Print and shaded views of the part. All mm, measured from the part's lowest x, y and z. Coordinates: 2 decimals unless noted, no trailing zeros. Loops run counter-clockwise (first coordinate to the right, second up) from the corner with the lowest first, then second, coordinate; pieces in that order, holes last. Notation, with made-up numbers: (8.25, 55) -> (18.25, 55) arc R29 ccw to (18.25, 77) -> close; hole circle Ø2 at (64.25, 44). An arc over 180 degrees is marked (long way). One line per item, written item: value. Start each with the question number.
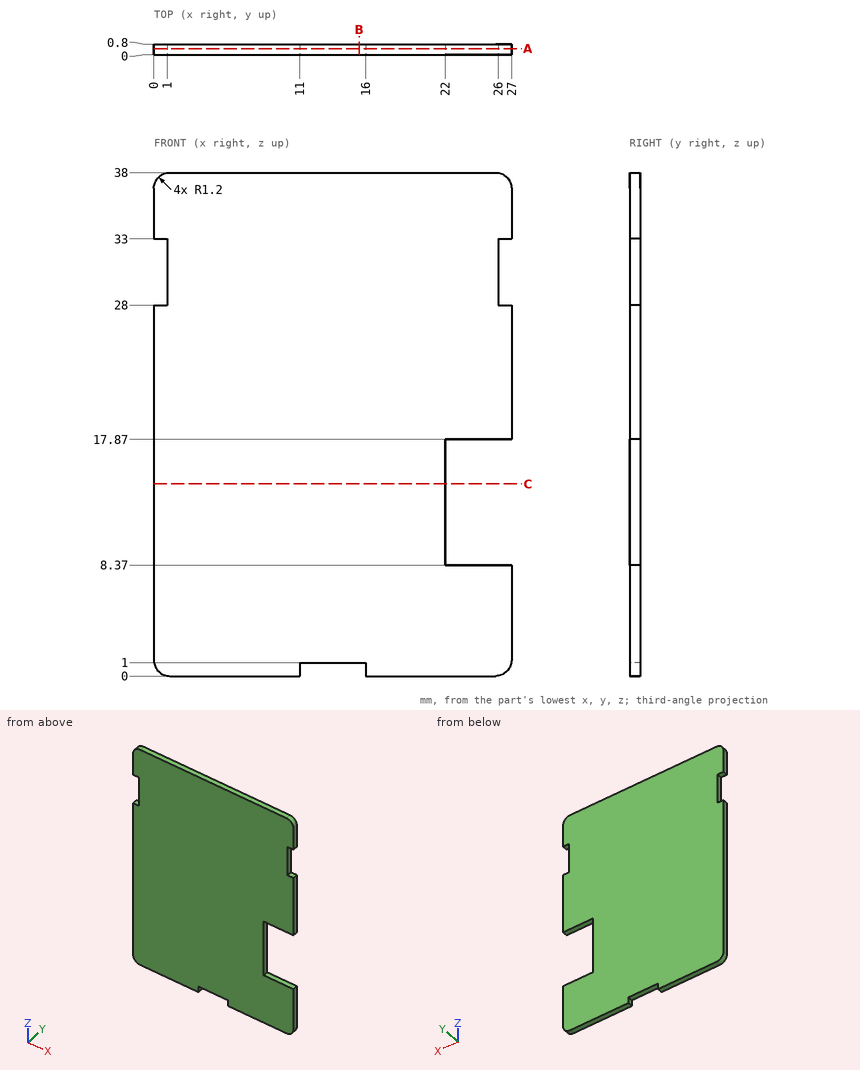
1) Slice it at C-C (z = 14.5). Give the cut face in (x, y).
2) Slice it at A-A (y = 0.45). Give the cut face in (x, z).
3) Slice it at B-B (x = 15.5). Give the cut face in (y, z), then the cut area to 3 significant figures.
4) Probe line 1 (Z direction, x = 24, y = 0.7); line 2 (Z direction, x = 12.5, y = 0.4); line 3 (X direction, y = 0.55, z = 32.5). List the from-to ranges inside material, lowest first. Write a range as from..to.
Check sheet entries:
1. outline: (0, 0) -> (22, 0) -> (22, 0.8) -> (0, 0.8) -> close
2. outline: (0, 1.2) arc R1.2 ccw to (1.2, 0) -> (11, 0) -> (11, 1) -> (16, 1) -> (16, 0) -> (25.8, 0) arc R1.2 ccw to (27, 1.2) -> (27, 8.37) -> (22, 8.37) -> (22, 17.87) -> (27, 17.87) -> (27, 28) -> (26, 28) -> (26, 33) -> (27, 33) -> (27, 36.8) arc R1.2 ccw to (25.8, 38) -> (1.2, 38) arc R1.2 ccw to (0, 36.8) -> (0, 33) -> (1, 33) -> (1, 28) -> (0, 28) -> close
3. outline: (0, 1) -> (0.8, 1) -> (0.8, 38) -> (0, 38) -> close
3. area: 29.6 mm^2
4. line 1: z = 0..8.37, 17.87..38
4. line 2: z = 1..38
4. line 3: x = 1..26
